Verification items for the finished model (mm, model axes). A direction names the side the tool comes from. Round coordinates to 2 decimals unless told otherwise and drop trailing zeros. Write each loop counter-clockwise with the first axis right and the second up, starting at its lowest first coordinate (ties: lowest second). Pieces come first, ordered by that corner, then holes. Notation, with made-up numbers: M 60.25,4 L 91.25,4 A17 ccw 91.25,24 Z; hole C 89.25,29.25 d1. An arc over 180 degrees is marked long. Answer in a Markdown table with one row per item. Add a question column.
1. Material ranges on probe 1 along Z at (x, y) = (-1.05, -21.5); probe 2 along Y at (x, z) = (-0.6, -6.5); probe 3 along Z at (x, y) = (-0.7, 26), recorded low to high.
2. Sectioned sample at A-A on y = -5.5. Record the cut outline in (x, z) (3 decimals), plus the area to 3 significant figures.
3. Set-up check for faces 1 (the flat face through (0.027, -35.36, -20.036)), 2 (the flat face through (0.03, -32.84, -19.32)): record each of +Z, -Z, +X, -X, +Y, -Y from which the full face is reachable in a straight line by a thin tool's end or side.
4. Sectioned sample at B-B on x = 1.15. Record the cut outline in (y, z).
5. Draft check along Z on faces 3 (the flat face through (0.027, 35.031, -20.604)), 4 (the flat face through (0.03, -33.15, 18.78)), 5 (the flat face through (0.027, -35.031, 20.604)). Enter one of: pulls with the +Z half, pulls with the -Z half, needs draft (parallel to the pull), parting line crosses it, or undercut.
6. Go/stop test with flat-tipped pins: pin 1 Ø1.5 at (x, z) = (1, 11) entering from -Y; pin 2 Ø1.5 at (x, z) = (0.5, 23) entering from -Y. Record where each tip stops, or that it passes through.
7. Sectioned sample at C-C on z = 12. Record the cut outline in (x, y) (3 decimals), plus the area to 3 significant figures.
```python
from build123d import *

# Parameters (mm, degrees)
F1_DEPTH = 1.905


with BuildPart() as f1:
    # F0 (on Right) → F1 (new body, symmetric)
    with BuildSketch(Plane.YZ):
        Polygon((-46.92703, 0), (-23.463515, -40.64), (23.463515, -40.64), (46.92703, 0), (23.463515, 40.64), (-23.463515, 40.64), align=None)
        Polygon((-43.994091, 0), (-21.997045, 38.1), (21.997045, 38.1), (43.994091, 0), (21.997045, -38.1), (-21.997045, -38.1), align=None, mode=Mode.SUBTRACT)
    extrude(amount=F1_DEPTH, both=True)


solid = f1.part
```
Geometry check:
| question | item | result |
|---|---|---|
| 1 | probe 1 | z = -40.64 to -38.1, 38.1 to 40.64 |
| 1 | probe 2 | y = -43.17 to -40.24, 40.24 to 43.17 |
| 1 | probe 3 | z = -36.25 to -31.17, 31.17 to 36.25 |
| 2 | outline | M -1.905,-40.64 L 1.905,-40.64 L 1.905,-38.1 L -1.905,-38.1 Z; M -1.905,38.1 L 1.905,38.1 L 1.905,40.64 L -1.905,40.64 Z |
| 2 | area | 19.4 mm2 |
| 3 | face 1 | -Z, +X, -X, -Y |
| 3 | face 2 | +X, -X |
| 4 | outline | M -46.93,0 L -23.46,-40.64 L 23.46,-40.64 L 46.93,0 L 23.46,40.64 L -23.46,40.64 Z; hole M -43.99,0 L -22,-38.1 L 22,-38.1 L 43.99,0 L 22,38.1 L -22,38.1 Z |
| 5 | face 3 | pulls with the -Z half |
| 5 | face 4 | undercut |
| 5 | face 5 | pulls with the +Z half |
| 6 | pin 1 | stops at y = -41.01 |
| 6 | pin 2 | stops at y = -34.08 |
| 7 | outline | M -1.905,-39.999 L 1.905,-39.999 L 1.905,-37.066 L -1.905,-37.066 Z; M -1.905,37.066 L 1.905,37.066 L 1.905,39.999 L -1.905,39.999 Z |
| 7 | area | 22.3 mm2 |
